Autodesk Inventor part; units mm, degrees
ref_plane "Work Plane1" through (22.5, 0, -31.25) normal (-1, 0, 0) x (0, 0, 1)
ref_plane "Work Plane2" through (41, 10, -1.55) normal (0, 0, -1) x (-1, 0, 0)
ref_plane "YZ Plane" through (0, 0, 0) normal (1, 0, 0) x (0, 1, 0)
sketch "Sketch1" plane through (0, 0, 0) normal (0, 1, 0) x (-1, 0, 0)
  line L0 (17.5, 31.25) -> (-17.5, 31.25)
  line L1 (-17.5, 31.25) -> (-17.5, -31.25)
  line L2 (-17.5, -31.25) -> (17.5, -31.25)
  line L3 (17.5, -31.25) -> (17.5, 31.25)
  line L4 (17.5, 31.25) -> (-17.5, -31.25) construction
  line L5 (-17.5, 31.25) -> (17.5, -31.25) construction
  point P0 (0, 0)
  dimension "d0" = 35
  dimension "d1" = 62.5
extrude "Extrusion1" add sketch "Sketch1" along normal blind 50
sketch "Sketch2" plane through (0, 50, 0) normal (0, 1, 0) x (1, 0, 0)
  line L0 (17.5, -31.25) -> (17.5, 31.25)
  line L1 (-17.5, -27.25) -> (17.5, -27.25)
  line L2 (17.5, -27.25) -> (17.5, 27.25)
  line L3 (17.5, 27.25) -> (-17.5, 27.25)
  line L4 (-17.5, 27.25) -> (-17.5, -27.25)
  line L5 (-17.5, -27.25) -> (17.5, 27.25) construction
  line L6 (17.5, -27.25) -> (-17.5, 27.25) construction
  line L7 (-17.5, -31.25) -> (17.5, -31.25)
  point P0 (0, 0)
  point P1 (17.5, -27.25)
  dimension "d4" = 4
extrude "Extrusion2" cut sketch "Sketch2" against normal blind 40
sketch "Sketch3" plane through (-17.5, 0, 31.25) normal (0, 0, 1) x (1, 0, 0)
  circle A0 centre (10, 31) radius 6.2
  line L0 (35, 10) -> (0, 10)
  line L1 (35, 10) -> (35, 50)
  line L2 (0, 0) -> (0, 50)
  point P0 (17.5, 0)
  point P1 (35, 30)
  dimension "d7" = 12.4
  dimension "d15" = 21
  dimension "d38" = 10
extrude "Extrusion3" cut sketch "Sketch3" against normal blind 8
sketch "Sketch4" plane through (17.5, 0, -31.25) normal (0, 0, -1) x (-1, 0, 0)
  circle A0 centre (25, 31) radius 6.2
  point P0 (17.5, 0)
extrude "Extrusion4" cut sketch "Sketch4" against normal blind 8
fillet "Fillet1" radius 2 2 edges at (0, 10, 27.25) (0, 10, -27.25)
sketch "Sketch5" plane through (17.5, 0, 31.25) normal (1, 0, 0) x (0, 0, -1)
  line L0 (4, 12) -> (4, 50)
  line L1 (0, 50) -> (4, 50)
  line L2 (0, 0) -> (0, 50)
  arc A0 (4, 12) -> (6, 10) centre (6, 12) ccw
  line L3 (0, 0) -> (62.5, 0)
  line L4 (56.5, 10) -> (6, 10)
  arc A1 (56.5, 10) -> (58.5, 12) centre (56.5, 12) ccw
  line L5 (58.5, 50) -> (58.5, 12)
  line L6 (62.5, 0) -> (62.5, 50)
  line L7 (58.5, 50) -> (62.5, 50)
  point P0 (31.25, 0)
extrude "Extrusion5" add sketch "Sketch5" along normal blind 30
sketch "Sketch6" plane through (0, 10, 0) normal (0, 1, 0) x (1, 0, 0)
  line L0 (5.7, 19.25) -> (41, 19.25)
  line L1 (41, 19.25) -> (41, -16.05)
  line L2 (41, -16.05) -> (5.7, -16.05)
  line L3 (5.7, -16.05) -> (5.7, 19.25)
  line L4 (5.7, 19.25) -> (41, -16.05) construction
  line L5 (41, 19.25) -> (5.7, -16.05) construction
  line L6 (-17.5, -25.25) -> (-17.5, 25.25)
  point P0 (0, 0)
  point P1 (23.35, 1.6)
  point P2 (-17.5, 0)
  point P3 (41, 1.6)
  point P4 (-17.5, 0)
  dimension "d16" = 35.3
  dimension "d17" = 35.3
  dimension "d84" = 1.6
  dimension "d108" = 58.5
extrude "Extrusion6" cut sketch "Sketch6" against normal blind 3
sketch "Sketch10" plane through (0, 0, 0) normal (0, -1, 0) x (1, 0, 0)
  line L0 (41, 16.05) -> (5.7, 16.05)
  line L1 (41, -19.25) -> (41, 16.05)
  line L2 (5.7, -19.25) -> (41, -19.25)
  line L3 (5.7, 16.05) -> (5.7, -19.25)
  point P0 (0, 0)
  point P1 (23.35, -14.25)
  point P2 (23.35, -19.25)
  dimension "d37" = 5
hole "Hole1" at (23.35, 0, -14.25) direction (0, 1, 0) diameter 3.1 end through all countersink diameter 4 countersink angle 90
ref_plane "Work Plane1" through (22.5, 0, -31.25) normal (-1, 0, 0) x (0, 0, 1)
fillet "Fillet4" radius 2 4 edges at (-17.5, 50, -29.25) (47.5, 50, -29.25) (47.5, 50, 29.25) (-17.5, 50, 29.25)
sketch "Sketch16" plane through (47.5, 0, -31.25) normal (0, 0, -1) x (-1, 0, 0)
  line L0 (63, 50) -> (2, 50)
  arc A0 (2, 50) -> (0, 48) centre (2, 48) ccw
  line L1 (0, 0) -> (0, 48)
  line L2 (0, 12) -> (65, 12)
  line L3 (40, 50) -> (40, 12)
  point P0 (47.5, 0)
  dimension "d93" = 40
extrude "Extrusion14" cut sketch "Sketch16" against normal blind 4
fillet "Fillet5" radius 2 1 edges at (7.5, 50, -29.25)
sketch "Sketch17" plane through (-17.5, 0, 31.25) normal (0, 0, 1) x (1, 0, 0)
  line L0 (2, 50) -> (63, 50)
  line L1 (65, 48) -> (65, 0)
  arc A0 (65, 48) -> (63, 50) centre (63, 48) ccw
  line L2 (0, 12) -> (65, 12)
  line L3 (25, 50) -> (25, 12)
  point P0 (17.5, 0)
  dimension "d88" = 40
extrude "Extrusion15" cut sketch "Sketch17" against normal blind 4
fillet "Fillet6" radius 2 2 edges at (47.5, 12, 29.25) (47.5, 12, -29.25)
fillet "Fillet7" radius 2 1 edges at (7.5, 50, 29.25)
ref_plane "Work Plane2" through (41, 10, -1.55) normal (0, 0, -1) x (-1, 0, 0)
mirror "Mirror5" about plane through (41, 10, -1.55) normal (0, 0, -1) of "Hole1"
chamfer "Chamfer1" distance 6 angle 45 1 edges at (-17.5, 0, 0)
sketch "Sketch18" plane through (5.5, 50, -31.25) normal (0, 0, -1) x (-1, 0, 0)
  line L0 (-37, -42.5) -> (-32, -42.5)
  line L1 (-32, -42.5) -> (-32, -47.5)
  line L2 (-32, -47.5) -> (-37, -47.5)
  line L3 (-37, -47.5) -> (-37, -42.5)
  line L4 (-42, -50) -> (-42, -40)
  point P0 (5.5, -50)
  point P1 (-42, -45)
  point P2 (-37, -45)
  point P3 (-42, -45)
  dimension "d98" = 5
  dimension "d99" = 5
  dimension "d100" = 5
extrude "Extrusion16" cut sketch "Sketch18" against normal blind 10
chamfer "Chamfer2" distance 1 angle 45 4 edges at (42.5, 7.5, -26.25) (37.5, 7.5, -26.25) (37.5, 2.5, -26.25) (42.5, 2.5, -26.25)
sketch "Sketch19" plane through (7.5, 12, 31.25) normal (0, 0, 1) x (1, 0, 0)
  line L0 (34, -4.5) -> (31, -4.5)
  line L1 (30, -5.5) -> (31, -4.5)
  line L2 (30, -5.5) -> (30, -8.5)
  line L3 (31, -9.5) -> (30, -8.5)
  line L4 (31, -9.5) -> (34, -9.5)
  line L5 (35, -8.5) -> (34, -9.5)
  line L6 (35, -8.5) -> (35, -5.5)
  line L7 (34, -4.5) -> (35, -5.5)
  point P0 (-7.5, -12)
extrude "Extrusion17" cut sketch "Sketch19" against normal blind 10
properties part number "base_engrane"
Part model, mm, in its own coordinate system. A direction names the side the tool comes from. Round coordinates to 2 decimals unless told otherwise and drop trailing zeros. Loops run counter-clockwise (first coordinate to the right, second up) from the corner with the lowest first, then second, coordinate; pieces in that order, holes last. Notation, with made-up numbers: (2, 15) -> (45, 15) arc R28 ccw to (45, 51) -> close; hole circle Ø9 at (-16.75, 86.5). An arc over 180 degrees is marked (long way). Use one line per item in the form item = value. Start each with the question number.
Item 1: Band-saw the part on C-C (x = 23.35). List the corners of the cut face in (y, z), plus the area to 3 significant figures.
Item 2: Band-saw the part on B-B (z = -14.25). List the corners of the cut face in (x, y).
Item 3: Band-saw the part on A-A (y = 31). List the corners of the cut face in (x, z).
Item 4: Tool access for faces 4 (the flat face through (27, 12, -29)), 5 (the cylindrical face through (14.55, 10.6, -26.68)), 6 (the flat face through (23, 7, -2)), 7 (the flat face through (42.5, 5, -26)), 8 (the flat face through (-14.5, 3, 0.4)): list every direction of +Z, -Z, +X, -X, +Y, -Y with a clear straight run to the whole face (end or side of a thin tool).
Item 5: Drop flat-ended pins along their axis: pin 1 Ø3 at (x, z) = (-9.5, 16) entering from +Y; pin 2 Ø10.5 at (x, z) = (23, -6.5) entering from +Y; pin 3 Ø1.5 at (y, z) = (5, -26) entering from -X; pin 4 Ø11 at (x, y) = (-7.5, 31) entering from -Z. Give the stop position or say it passes through.
Item 6: Drill centre lines: line 1 along Z through (x, y) = (23.35, 2.5); line 2 along Z through (x, y) = (3, 42); line 3 along Y through (x, z) = (-7.5, -28.1). Where is each one in solid material? Low to high.
Item 7: Two-plate mould, pull along Y, no slides. Class faces 1 (the flat face through (40, 7.5, 26)), 2 (the cylindrical face through (46.9, 11.43, 28.89)), 3 (the flat face through (7, 19, 31.25)): released by +Y, released by -Y, zero draft, split by the parting line, or undercut.
Item 8: Band-saw the part on D-D (y = 20). List the corners of the cut face in (x, z), plus the area to 3 significant figures.
Data:
q1.outline = (0, -31.25) -> (12, -31.25) -> (12, -27.25) arc R2 cw to (10, -25.25) -> (10, -19.25) -> (7, -19.25) -> (7, -15.8) -> (0.45, -15.8) -> (0, -16.25) -> close; (0, -12.25) -> (0.45, -12.7) -> (7, -12.7) -> (7, 9.6) -> (0.45, 9.6) -> (0, 9.15) -> close; (0, 13.15) -> (0.45, 12.7) -> (7, 12.7) -> (7, 16.05) -> (10, 16.05) -> (10, 25.25) arc R2 cw to (12, 27.25) -> (12, 31.25) -> (0, 31.25) -> close
q1.area = 493 mm^2
q2.outline = (-17.5, 6) -> (-11.5, 0) -> (21.35, 0) -> (21.8, 0.45) -> (21.8, 7) -> (5.7, 7) -> (5.7, 10) -> (-17.5, 10) -> close; (24.9, 0.45) -> (25.35, 0) -> (47.5, 0) -> (47.5, 10) -> (41, 10) -> (41, 7) -> (24.9, 7) -> close
q3.outline = (-17.5, -31.25) -> (-13.7, -31.25) -> (-13.7, -27.25) -> (-17.5, -27.25) -> close; (-17.5, 27.25) -> (-13.7, 27.25) -> (-13.7, 31.25) -> (-17.5, 31.25) -> close; (-1.3, -31.25) -> (7.5, -31.25) -> (7.5, -27.25) -> (-1.3, -27.25) -> close; (-1.3, 27.25) -> (7.5, 27.25) -> (7.5, 31.25) -> (-1.3, 31.25) -> close
q4.face_4 = +Z, -Z, +X, +Y
q4.face_5 = +X, -X, +Y
q4.face_6 = +Y
q4.face_7 = -Z
q4.face_8 = +Z, -Z, -X, -Y
q5.pin_1 = 10
q5.pin_2 = 7
q5.pin_3 = -17.25
q5.pin_4 = through
q6.line_1 = -31.25 to -15.8, -12.7 to 9.6, 12.7 to 31.25
q6.line_2 = -31.25 to -27.25, 27.25 to 31.25
q6.line_3 = 0 to 24.8, 37.2 to 50
q7.face_1 = undercut
q7.face_2 = released by +Y
q7.face_3 = zero draft
q8.outline = (-17.5, -31.25) -> (7.5, -31.25) -> (7.5, -27.25) -> (-17.5, -27.25) -> close; (-17.5, 27.25) -> (7.5, 27.25) -> (7.5, 31.25) -> (-17.5, 31.25) -> close
q8.area = 200 mm^2
